Source: CAD feature listing. Evaluate the final solid. Frame: model axes, mm. A direction names the side the tool comes from. Coordinates: 2 decimals unless noted, no trailing zeros. Write each loop counter-clockwise with the first axis right and the second up, starting at its lowest first coordinate (ties: lowest second). Pieces come first, ordered by that corner, then holes. Notation, with made-up numbers: M 3,57.5 L 38,57.5 A28 cw 38,88.5 Z; hole C -1,18 d10. An arc over 180 degrees is marked long. One line per item, written item: value. Start each with the question number.
Item 1: Pin query (flat end, axial travel): P1, Ø5, axis at y = -13.5, z = 4, coming from the -X side; P2, Ø8, axis at x = -40, z = 0, coming from the +Y side; P3, Ø5.5, axis at y = 4.5, z = 2.5, coming from the +X side; P4, Ø1, axis at x = 6.5, z = -7.5, coming from the +Y side. Return the tip coordinate at first contact, or that it passes through.
Item 2: Cut plane B-B, the plane x = 25.5. Output: boundary loops of the cut face in (y, z), then the cut area to 3 significant figures.
Item 3: Cut plane A-A, the plane y = 29. Output: boundary loops of the cut face in (x, z).
Item 4: Cut plane C-C, the plane y = -33. Output: boundary loops of the cut face in (x, z), then the cut area to 3 significant figures.
Item 5: Mould query, pull axis X, two halves, no side actions, for faces 1 (the cylindrical face through (-0.069, -24.334, -0.14)), 2 (the flat face through (-50, 33, 0)), 3 (the flat face through (45, -27, 2)). Classes: released by +X, released by -X, zero draft, split by the parting line, or undercut.
Item 6: Ray query, L1, parallel to Z at x = -40, y = -33.25; L2, parallel to Y at x = 35.5, z = 5; L3, parallel to X at y = -30.5, z = 0. Return the intervals inside material, ascending. Write a range as from..to.
Item 7: Set-up query: faces 4 (the cylindrical face through (-11.26, -14.2, -0.14)), 5 (the flat face through (-17.53, 32.35, 0.14)), 6 (the flat face through (45, 27, -2)), 7 (the flat face through (-17.176, -32.16, 0.14)). Return all of +Z, -Z, +X, -X, +Y, -Y with unobstructed straight access to the full face (end or side cutting, diameter ignored); none if empty.
```python
from build123d import *

# Parameters (mm, degrees)
BOSS_EXTRUDE1_DEPTH                        = 10
FILLET1_R                                  = 10
F_10_0MM_DOWEL_HOLE1_D                     = 10
F_10_0MM_DOWEL_HOLE1_DEPTH                 = 24.5
F_10_0MM_DOWEL_HOLE1_CSINK_D               = 10.05
F_10_0MM_DOWEL_HOLE1_CSINK_ANGLE           = 90
F_10_0MM_DOWEL_HOLE1_TIP                   = 3.004303095
F_10_0MM_DOWEL_HOLE1_ON_FACE_2_D           = 10
F_10_0MM_DOWEL_HOLE1_ON_FACE_2_DEPTH       = 24.5
F_10_0MM_DOWEL_HOLE1_ON_FACE_2_CSINK_D     = 10.05
F_10_0MM_DOWEL_HOLE1_ON_FACE_2_CSINK_ANGLE = 90
F_10_0MM_DOWEL_HOLE1_ON_FACE_2_TIP         = 3.004303095
FILLET2_R                                  = 3


with BuildPart() as part:
    # Sketch1 → Boss-Extrude1 (new, symmetric)
    with BuildSketch(Plane.XY):
        Polygon((-50, 27), (-50, 39), (-30, 39), (0, 23), (30, 39), (50, 39), (50, 27), (30, 27), (10, 15), (10, -15), (30, -27), (50, -27), (50, -39), (30, -39), (0, -23), (-30, -39), (-50, -39), (-50, -27), (-30, -27), (-10, -15), (-10, 15), (-30, 27), align=None)
    extrude(amount=BOSS_EXTRUDE1_DEPTH, both=True)

    # Fillet1
    fillet1_edges = [part.edges().sort_by_distance(p)[0] for p in [
        (-10, 15, 0),
        (0, 23, 0),
        (10, 15, 0),
        (10, -15, 0),
        (0, -23, 0),
        (-10, -15, 0),
    ]]
    fillet(fillet1_edges, radius=FILLET1_R)

    # Ø10.0mm Dowel Hole1
    with Locations(Plane(origin=(-40, 39, 0), x_dir=(1, 0, 0), z_dir=(0, 1, 0))):
        with Locations((0, 0), (80, 0)):
            CounterSinkHole(F_10_0MM_DOWEL_HOLE1_D / 2, F_10_0MM_DOWEL_HOLE1_CSINK_D / 2, depth=F_10_0MM_DOWEL_HOLE1_DEPTH, counter_sink_angle=F_10_0MM_DOWEL_HOLE1_CSINK_ANGLE)
            with Locations((0, 0, -(F_10_0MM_DOWEL_HOLE1_DEPTH + F_10_0MM_DOWEL_HOLE1_TIP / 2))):  # 118° drill point
                Cone(0, F_10_0MM_DOWEL_HOLE1_D / 2, F_10_0MM_DOWEL_HOLE1_TIP, mode=Mode.SUBTRACT)

    # Ø10.0mm Dowel Hole1 on face 2
    with Locations(Plane(origin=(-40, -27, 0), x_dir=(0, 0, 1), z_dir=(0, 1, 0))):
        with Locations((0, 0), (0, 80)):
            CounterSinkHole(F_10_0MM_DOWEL_HOLE1_ON_FACE_2_D / 2, F_10_0MM_DOWEL_HOLE1_ON_FACE_2_CSINK_D / 2, depth=F_10_0MM_DOWEL_HOLE1_ON_FACE_2_DEPTH, counter_sink_angle=F_10_0MM_DOWEL_HOLE1_ON_FACE_2_CSINK_ANGLE)
            with Locations((0, 0, -(F_10_0MM_DOWEL_HOLE1_ON_FACE_2_DEPTH + F_10_0MM_DOWEL_HOLE1_ON_FACE_2_TIP / 2))):  # 118° drill point
                Cone(0, F_10_0MM_DOWEL_HOLE1_ON_FACE_2_D / 2, F_10_0MM_DOWEL_HOLE1_ON_FACE_2_TIP, mode=Mode.SUBTRACT)

    # Fillet2
    fillet2_edges = [part.edges().sort_by_distance(p)[0] for p in [
        (-30, 27, 0),
        (30, 27, 0),
        (30, -27, 0),
        (-30, -27, 0),
    ]]
    fillet(fillet2_edges, radius=FILLET2_R)


solid = part.part
```
From the geometry:
1. P1: stops at x = -12.54
1. P2: passes through
1. P3: stops at x = 10
1. P4: stops at y = 26.73
2. outline: M -36.6,-10 L -24.3,-10 L -24.3,10 L -36.6,10 Z; M 24.3,-10 L 36.6,-10 L 36.6,10 L 24.3,10 Z
2. area: 492 mm²
3. outline: M -50,-10 L -11.25,-10 L -11.25,10 L -50,10 Z; M 11.25,-10 L 50,-10 L 50,10 L 11.25,10 Z; hole C -40,0 d10; hole C 40,0 d10
4. outline: M -50,-10 L -18.75,-10 L -18.75,10 L -50,10 Z; M 18.75,-10 L 50,-10 L 50,10 L 18.75,10 Z; hole C -40,0 d10; hole C 40,0 d10
4. area: 1,090 mm²
5. face 1: undercut
5. face 2: released by -X
5. face 3: zero draft
6. L1: z = -10..-5, 5..10
6. L2: y = -39..-27, 27..39
6. L3: x = -50..-45, -35..-14.06, 14.06..35, 45..50
7. face 4: +Z, -Z, -X
7. face 5: +Z, -Z, +Y
7. face 6: +Z, -Z, +X
7. face 7: +Z, -Z, -Y
